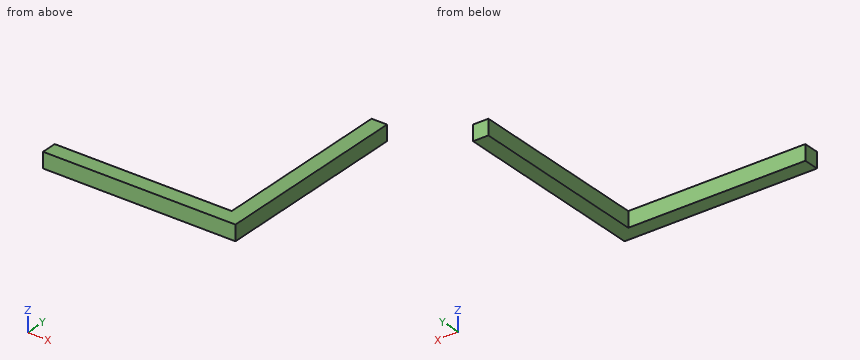
```python
from build123d import *

# Parameters (mm, degrees)
ESQUISSE1_W        = 115
ESQUISSE1_H        = 10
BOSS_EXTRU_1_DEPTH = 10
ESQUISSE2_W        = 10
ESQUISSE2_H        = 130
BOSS_EXTRU_2_DEPTH = 10


with BuildPart() as part:
    # Esquisse1 → Boss.-Extru.1 (new body)
    with BuildSketch(Plane.XY):
        with Locations((39.062768353, 9.317091479)):
            Rectangle(ESQUISSE1_W, ESQUISSE1_H)
    extrude(amount=BOSS_EXTRU_1_DEPTH)

    # Esquisse2 → Boss.-Extru.2 (add)
    with BuildSketch(Plane(origin=(96.562768353, 0, 0), x_dir=(0, 0, -1), z_dir=(1, 0, 0))):
        with Locations((-5, 69.317091479)):
            Rectangle(ESQUISSE2_W, ESQUISSE2_H)
    extrude(amount=BOSS_EXTRU_2_DEPTH)


solid = part.part
```
The listing builds one solid part. Answer for the finished solid, in the listing's coordinates (mm). Coordinates: 2 decimals unless noted, no trailing zeros. Write each loop counter-clockwise with the first axis right and the second up, starting at its lowest first coordinate (ties: lowest second). Pieces come first, ordered by that corner, then holes. Notation, with made-up numbers: (-27.5, -2.5) -> (-19.5, -2.5) arc R21 ccw to (-19.5, 25.5) -> close; hole circle Ø9 at (65.5, -35). An arc over 180 degrees is marked (long way). Write each question's results on one line, items separated by ' | '. Start each with the question number.
1) A cutting plane is placed at C-C (z = 6.5). Determine the outline of the cut face in (x, y), then the cut area to 3 significant figures.
2) Flat-ended cylindrical pins translate along their axes: pin 1 Ø2 at (x, z) = (36, 7.5) entering from +Y; pin 2 Ø5 at (y, z) = (118.5, 4.5) entering from -X. Find the tip coordinate at first contact, or state that the pin passes through.
3) A cutting plane is placed at A-A (y = 81.5). Determine the outline of the cut face in (x, z), then the cut area to 3 significant figures.
4) Straight lines are drawn through the part: probe 1 along Y at (x, z) = (34, 4.75); probe 2 along X at (y, z) = (55, 7.5). For each, find the intervals that lie inside material, in ascending order.
5) A cutting plane is placed at B-B (x = 31.5). Determine the outline of the cut face in (y, z), then the cut area to 3 significant figures.
Values follow:
1) outline: (-18.44, 4.32) -> (106.56, 4.32) -> (106.56, 134.32) -> (96.56, 134.32) -> (96.56, 14.32) -> (-18.44, 14.32) -> close | area: 2,450 mm²
2) pin 1: y = 14.32 | pin 2: x = 96.56
3) outline: (96.56, 0) -> (106.56, 0) -> (106.56, 10) -> (96.56, 10) -> close | area: 100 mm²
4) probe 1: 4.32 to 14.32 | probe 2: 96.56 to 106.56
5) outline: (4.32, 0) -> (14.32, 0) -> (14.32, 10) -> (4.32, 10) -> close | area: 100 mm²
